Model file for the job. Use its own axes, mm. Face numbers are marked on the shaded views. Coordinates: 2 decimals unless noted, no trailing zeros. Loops run counter-clockwise (first coordinate to the right, second up) from the corner with the lowest first, then second, coordinate; pieces in that order, holes last. Notation, with made-up numbers: (25.5, 53) -> (82.5, 53) arc R27 cw to (82.5, 78) -> close; hole circle Ø11 at (14.25, 69). An arc over 180 degrees is marked (long way). Use one line per item in the form item = value.
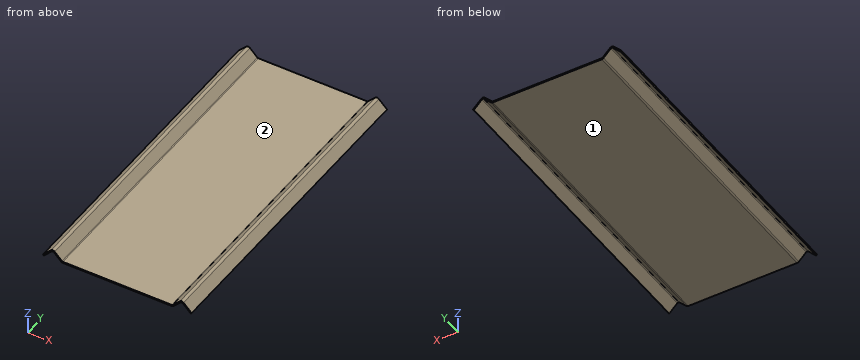
```python
from build123d import *

# Parameters (mm, degrees)
F1_DEPTH = 1000
F2_R     = 4
F3_R     = 8


with BuildPart() as f1:
    # F0 (on Front) → F1 (new body)
    with BuildSketch(Plane.XZ):
        Polygon((-175, 0), (0, 0), (175, 0), (203.284271, 28.284271), (231.568542, 0), (234.39697, 2.828427), (203.284271, 33.941125), (173.343146, 4), (0, 4), (-173.343146, 4), (-203.284271, 33.941125), (-234.39697, 2.828427), (-231.568542, 0), (-203.284271, 28.284271), align=None)
    extrude(amount=-F1_DEPTH)

    # F2
    f2_edges = [f1.edges().sort_by_distance(p)[0] for p in [
        (-203.284271, 500, 28.284271),
        (203.284271, 500, 28.284271),
        (-173.343146, 500, 4),
        (173.343146, 500, 4),
    ]]
    fillet(f2_edges, radius=F2_R)

    # F3
    f3_edges = [f1.edges().sort_by_distance(p)[0] for p in [
        (-203.284271, 500, 33.941125),
        (203.284271, 500, 33.941125),
        (-175, 500, 0),
        (175, 500, 0),
    ]]
    fillet(f3_edges, radius=F3_R)


solid = f1.part
```
Q1. Pin check, flat tips, straight feed: pin 1 Ø4 at (x, y) = (-34.5, 649) entering from +Z; pin 2 Ø6 at (y, z) = (383, 25) entering from +X; pin 3 Ø5 at (y, z) = (398, 10) entering from -X. Stop position of each tip, or through.
Result:
pin_1 = 4
pin_2 = 215.23
pin_3 = -229.73
Q2. Band-saw the part on A-A, the plane y = 696. Write the cut outline in (x, z), and give its area (3 significant figures).
Result:
outline = (-234.4, 2.83) -> (-231.57, 0) -> (-206.11, 25.46) arc R4 cw to (-200.46, 25.46) -> (-177.34, 2.34) arc R8 ccw to (-171.69, 0) -> (171.69, 0) arc R8 ccw to (177.34, 2.34) -> (200.46, 25.46) arc R4 cw to (206.11, 25.46) -> (231.57, 0) -> (234.4, 2.83) -> (208.94, 28.28) arc R8 ccw to (197.63, 28.28) -> (174.51, 5.17) arc R4 cw to (171.69, 4) -> (-171.69, 4) arc R4 cw to (-174.51, 5.17) -> (-197.63, 28.28) arc R8 ccw to (-208.94, 28.28) -> close
area = 2,040 mm2
Q3. Wall check: line 1 along X through (y, z) = (414.5, 14); line 2 along X through (y, z) = (139, 2); line 3 along X through (y, z) = (295.5, 26). Give the ranges that are in metal, low to high.
Result:
line_1 = -223.23 to -217.57, -189 to -183.34, 183.34 to 189, 217.57 to 223.23
line_2 = -233.57 to -229.57, -176.98 to 176.98, 229.57 to 233.57
line_3 = -211.23 to -205.44, -201.13 to -195.34, 195.34 to 201.13, 205.44 to 211.23
Q4. Band-saw the part on C-C, the plane x = 14. Write the cut outline in (y, z), and give its area (3 significant figures).
Result:
outline = (0, 0) -> (1000, 0) -> (1000, 4) -> (0, 4) -> close
area = 4,000 mm2
Q5. Band-saw the part on B-B, the plane z = 13. Write the cut outline in (x, y).
Result:
outline = (-224.23, 0) -> (-218.57, 0) -> (-218.57, 1000) -> (-224.23, 1000) -> close; (-188, 0) -> (-182.34, 0) -> (-182.34, 1000) -> (-188, 1000) -> close; (182.34, 0) -> (188, 0) -> (188, 1000) -> (182.34, 1000) -> close; (218.57, 0) -> (224.23, 0) -> (224.23, 1000) -> (218.57, 1000) -> close
Q6. Mould opens along X. For the marked faces 1 and 2 say: released by +X, released by -X, zero draft, split by the parting line, or undercut.
Result:
face_1 = zero draft
face_2 = undercut
